Check sheet for the modelled part. Datum: model origin and axes. Units: mm. Coordinates: 2 decimals unless noted, no trailing zeros. Order: outer loops, then holes, each group sorted by start corner. A loop starts at its lowest first (then second) coordinate and runs counter-clockwise, first axis right, second up.
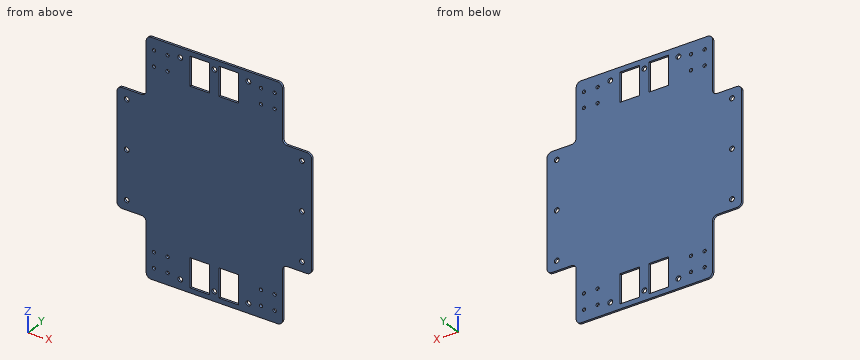
from build123d import *

# Parameters (mm, degrees)
SKETCH_1_R          = 1.7
SKETCH_1_R_2        = 2.5
SKETCH_1_W          = 20
SKETCH_1_H          = 30
EXTRUDE_6_DEPTH     = 2
SKETCH_2_W          = 30
SKETCH_2_H          = 10
CUT_EXTRUDE_2_DEPTH = 2


with BuildPart() as part:
    # 草图1 → 凸台-拉伸6 (new body)
    with BuildSketch(Plane(origin=(0, 0, 0), x_dir=(1, 0, 0), z_dir=(0, 1, 0))):
        with BuildLine():
            Line((-75, 80), (-95, 80))
            ThreePointArc((-95, 80), (-98.535533906, 78.535533906), (-100, 75))
            Line((-100, 75), (-100, -75))
            ThreePointArc((-100, -75), (-98.535533906, -78.535533906), (-95, -80))
            Line((-95, -80), (-75, -80))
            ThreePointArc((-75, -80), (-71.464466094, -81.464466094), (-70, -85))
            Line((-70, -85), (-70, -115))
            ThreePointArc((-70, -115), (-68.535533906, -118.535533906), (-65, -120))
            Line((-65, -120), (65, -120))
            ThreePointArc((65, -120), (68.535533906, -118.535533906), (70, -115))
            Line((70, -115), (70, -85))
            ThreePointArc((70, -85), (71.464466094, -81.464466094), (75, -80))
            Line((75, -80), (95, -80))
            ThreePointArc((95, -80), (98.535533906, -78.535533906), (100, -75))
            Line((100, -75), (100, 75))
            ThreePointArc((100, 75), (98.535533906, 78.535533906), (95, 80))
            Line((95, 80), (75, 80))
            ThreePointArc((75, 80), (71.464466094, 81.464466094), (70, 85))
            Line((70, 85), (70, 115))
            ThreePointArc((70, 115), (68.535533906, 118.535533906), (65, 120))
            Line((65, 120), (-65, 120))
            ThreePointArc((-65, 120), (-68.535533906, 118.535533906), (-70, 115))
            Line((-70, 115), (-70, 85))
            ThreePointArc((-70, 85), (-71.464466094, 81.464466094), (-75, 80))
        make_face()
        with Locations(Location((-62, -108, 0), (0, 0, 270))):
            Circle(SKETCH_1_R, mode=Mode.SUBTRACT)
        with Locations(Location((-48, -108, 0), (0, 0, 270))):
            Circle(SKETCH_1_R, mode=Mode.SUBTRACT)
        with Locations(Location((-62, -92, 0), (0, 0, 270))):
            Circle(SKETCH_1_R, mode=Mode.SUBTRACT)
        with Locations(Location((-48, -92, 0), (0, 0, 270))):
            Circle(SKETCH_1_R, mode=Mode.SUBTRACT)
        with Locations(Location((-35, -110, 0), (0, 0, 270))):
            Circle(SKETCH_1_R_2, mode=Mode.SUBTRACT)
        with Locations((-15, -100)):
            Rectangle(SKETCH_1_W, SKETCH_1_H, mode=Mode.SUBTRACT)
        with Locations(Location((-90, -50, 0), (0, 0, 270))):
            Circle(SKETCH_1_R_2, mode=Mode.SUBTRACT)
        with Locations(Location((0, -110, 0), (0, 0, 270))):
            Circle(SKETCH_1_R_2, mode=Mode.SUBTRACT)
        with Locations((15, -100)):
            Rectangle(SKETCH_1_W, SKETCH_1_H, mode=Mode.SUBTRACT)
        with Locations(Location((35, -110, 0), (0, 0, 270))):
            Circle(SKETCH_1_R_2, mode=Mode.SUBTRACT)
        with Locations(Location((48, -108, 0), (0, 0, 270))):
            Circle(SKETCH_1_R, mode=Mode.SUBTRACT)
        with Locations(Location((62, -108, 0), (0, 0, 270))):
            Circle(SKETCH_1_R, mode=Mode.SUBTRACT)
        with Locations(Location((48, -92, 0), (0, 0, 270))):
            Circle(SKETCH_1_R, mode=Mode.SUBTRACT)
        with Locations(Location((62, -92, 0), (0, 0, 270))):
            Circle(SKETCH_1_R, mode=Mode.SUBTRACT)
        with Locations(Location((90, -50, 0), (0, 0, 270))):
            Circle(SKETCH_1_R_2, mode=Mode.SUBTRACT)
        with Locations(Location((-90, 0, 0), (0, 0, 270))):
            Circle(SKETCH_1_R_2, mode=Mode.SUBTRACT)
        with Locations(Location((-90, 50, 0), (0, 0, 270))):
            Circle(SKETCH_1_R_2, mode=Mode.SUBTRACT)
        with Locations(Location((-62, 92, 0), (0, 0, 270))):
            Circle(SKETCH_1_R, mode=Mode.SUBTRACT)
        with Locations(Location((-62, 108, 0), (0, 0, 270))):
            Circle(SKETCH_1_R, mode=Mode.SUBTRACT)
        with Locations(Location((-48, 108, 0), (0, 0, 270))):
            Circle(SKETCH_1_R, mode=Mode.SUBTRACT)
        with Locations(Location((-48, 92, 0), (0, 0, 270))):
            Circle(SKETCH_1_R, mode=Mode.SUBTRACT)
        with Locations(Location((-35, 110, 0), (0, 0, 270))):
            Circle(SKETCH_1_R_2, mode=Mode.SUBTRACT)
        Polygon((-5, 115), (-5, 100), (-5, 85), (-25, 85), (-25, 115), align=None, mode=Mode.SUBTRACT)
        with Locations(Location((90, 0, 0), (0, 0, 270))):
            Circle(SKETCH_1_R_2, mode=Mode.SUBTRACT)
        with Locations(Location((90, 50, 0), (0, 0, 270))):
            Circle(SKETCH_1_R_2, mode=Mode.SUBTRACT)
        with Locations((15, 100)):
            Rectangle(SKETCH_1_W, SKETCH_1_H, mode=Mode.SUBTRACT)
        with Locations(Location((0, 110, 0), (0, 0, 270))):
            Circle(SKETCH_1_R_2, mode=Mode.SUBTRACT)
        with Locations(Location((35, 110, 0), (0, 0, 270))):
            Circle(SKETCH_1_R_2, mode=Mode.SUBTRACT)
        with Locations(Location((48, 92, 0), (0, 0, 270))):
            Circle(SKETCH_1_R, mode=Mode.SUBTRACT)
        with Locations(Location((62, 92, 0), (0, 0, 270))):
            Circle(SKETCH_1_R, mode=Mode.SUBTRACT)
        with Locations(Location((48, 108, 0), (0, 0, 270))):
            Circle(SKETCH_1_R, mode=Mode.SUBTRACT)
        with Locations(Location((62, 108, 0), (0, 0, 270))):
            Circle(SKETCH_1_R, mode=Mode.SUBTRACT)
    extrude(amount=EXTRUDE_6_DEPTH)

    # 草图2 → 切除-拉伸2 (cut)
    with BuildSketch(Plane(origin=(0, 2, 0), x_dir=(1, 0, 0), z_dir=(0, 1, 0))):
        with BuildLine():
            Line((-70, 75), (-100, 75))
            Line((-100, 75), (-100, 60))
            Line((-100, 60), (-95, 60))
            Line((-95, 60), (-75, 60))
            ThreePointArc((-75, 60), (-71.464466094, 61.464466094), (-70, 65))
            Line((-70, 65), (-70, 75))
        make_face()
        with BuildLine():
            Line((-100, 60), (-100, 55))
            ThreePointArc((-100, 55), (-98.535533906, 58.535533906), (-95, 60))
            Line((-95, 60), (-100, 60))
        make_face()
        with Locations((-85, 80)):
            Rectangle(SKETCH_2_W, SKETCH_2_H)
        with BuildLine():
            Line((100, 55), (100, 60))
            Line((100, 60), (95, 60))
            ThreePointArc((95, 60), (98.535533906, 58.535533906), (100, 55))
        make_face()
        with BuildLine():
            ThreePointArc((75, 60), (71.464466094, 61.464466094), (70, 65))
            Line((70, 65), (70, 75))
            Line((70, 75), (100, 75))
            Line((100, 75), (100, 60))
            Line((100, 60), (75, 60))
        make_face()
        with Locations((85, 80)):
            Rectangle(SKETCH_2_W, SKETCH_2_H)
        with BuildLine():
            ThreePointArc((100, -55), (98.535533906, -58.535533906), (95, -60))
            Line((95, -60), (75, -60))
            ThreePointArc((75, -60), (71.464466094, -61.464466094), (70, -65))
            Line((70, -65), (70, -75))
            Line((70, -75), (100, -75))
            Line((100, -75), (100, -60))
            Line((100, -60), (100, -55))
        make_face()
        with Locations((85, -80)):
            Rectangle(SKETCH_2_W, SKETCH_2_H)
        with Locations((-85, -80)):
            Rectangle(SKETCH_2_W, SKETCH_2_H)
        with BuildLine():
            ThreePointArc((-100, -55), (-98.535533906, -58.535533906), (-95, -60))
            Line((-95, -60), (-75, -60))
            ThreePointArc((-75, -60), (-71.464466094, -61.464466094), (-70, -65))
            Line((-70, -65), (-70, -75))
            Line((-70, -75), (-100, -75))
            Line((-100, -75), (-100, -60))
            Line((-100, -60), (-100, -55))
        make_face()
    extrude(amount=-CUT_EXTRUDE_2_DEPTH, mode=Mode.SUBTRACT)


solid = part.part
(1) Cross-section at C-C (y = 0.6). Count the separate pieces of the cut face and the enclosed holes in it, and give its area (3 significant figures).
Filled in:
separate pieces: 1
enclosed holes: 32
area: 38,000 mm2
(2) Cross-section at A-A (z = 50). Enter the section's corners in (x, y).
Filled in:
outline: (-100, 0) - (-92.5, 0) - (-92.5, 2) - (-100, 2) - close; (-87.5, 0) - (87.5, 0) - (87.5, 2) - (-87.5, 2) - close; (92.5, 0) - (100, 0) - (100, 2) - (92.5, 2) - close
(3) Go/stop test with flat-tipped pins: P1, Ø1, axis at y = 0.5, z = -83.5, coming from the +X side; P2, Ø3, axis at x = -62, z = -92, coming from the +Y side; P3, Ø1, axis at y = 1, z = -96, coming from the -X side. Record where each tip stops, or that it passes through.
Filled in:
P1: stops at x = 70
P2: passes through
P3: stops at x = -70
(4) Thickness scan on probe 1 along Z at (x, y) = (-15, 1.75); probe 2 along X at (y, z) = (0.55, 110); probe 3 along X at (y, z) = (0.45, -75.5). Record the ranges inside material, lowest first.
Filled in:
probe 1: z = -120 to -115, -85 to 85, 115 to 120
probe 2: x = -70 to -37.5, -32.5 to -25, -5 to -2.5, 2.5 to 5, 25 to 32.5, 37.5 to 70
probe 3: x = -70 to 70
(5) Cross-section at B-B (x = -8). Enter the section's corners in (y, z), and give its area (3 significant figures).
Filled in:
outline: (0, -120) - (2, -120) - (2, -115) - (0, -115) - close; (0, -85) - (2, -85) - (2, 85) - (0, 85) - close; (0, 115) - (2, 115) - (2, 120) - (0, 120) - close
area: 360 mm2
